Read the model definition and answer for the solid it produces. Units are mm, in the model's axes. A direction names the side the tool comes from. Round coordinates to 2 decimals unless told otherwise and drop trailing zeros. Order: outer loops, then holes, each group sorted by start corner. A loop starts at its lowest first (then second) coordinate and runs counter-clockwise, first axis right, second up. Notation, with made-up numbers: (38, -38.5) - (58, -38.5) arc R17 ccw to (58, -28.5) - close; hole circle Ø3 at (14.5, 23). An arc over 180 degrees is marked (long way). One line per question, with ' | ' between items. Start each with the question number.
1) For faces 1 (the flat face through (0, 1, 0)), 2 (the flat face through (14, -37, 12)), determine the directions among +Z, -Z, +X, -X, +Y, -Y from which every point of the face is accessible in a straight line to the end or side of a thin tool.
2) The part is cut by section D-D, the plane z = 20. Count the separate pieces of the cut face and the enclosed holes in it, plus the area to 3 significant figures.
3) Straight lines are drawn through the part: line 1 (Y direction, x = 16.5, z = 17.25); line 2 (X direction, y = -36.5, z = 6.5); line 3 (Y direction, x = -17.5, z = 22.5). For each, find the intervals that lie inside material, in ascending order. Write a range as from..to.
4) Flat-ended cylindrical pins translate along their axes: pin 1 (4 mm diameter, centred on x = -6.5, y = -4, fed in from +Z); pin 2 (1.2 mm diameter, centred on x = -16.5, y = -36, fed in from +Z). Find the tip coordinate at first contact, or state that the pin passes through.
5) The part is cut by section C-C, the plane y = 36.5. Give the vertices of the cut face in (x, z).
6) The part is cut by section B-B, the plane x = 0. Give the vertices of the cut face in (y, z), plus the area to 3 significant figures.
7) The mould has two halves that part along X. Classify faces 3 (the flat face through (-20, -1, 12)), 4 (the flat face through (-19.4, 0.2, 25)), 5 (the flat face through (16, 38, 23)): pulls with the +X half, pulls with the -X half, needs draft (parallel to the pull), parting line crosses it, or undercut.
8) The part is cut by section A-A, the plane z = 4.75. Give the vertices of the cut face in (x, y).
from build123d import *

# Parameters (mm, degrees)
F0_W     = 40
F0_H     = 80
F1_DEPTH = 25
F2_T     = -1
F3_W     = 5
F3_H     = 5
F3_R     = 0.75
F3_W_2   = 3
F3_H_2   = 1
F4_DEPTH = 22
F6_DEPTH = 25


with BuildPart() as f1:
    # F0 (on Top) → F1 (new body)
    with BuildSketch(Plane.XY):
        Rectangle(F0_W, F0_H)
    extrude(amount=F1_DEPTH)

    # F2
    f2_openings = [f1.faces().sort_by_distance(p)[0] for p in [
        (0, 0, 25),
    ]]
    offset(amount=F2_T, openings=f2_openings)

    # F3 (on face) → F4 (join)
    with BuildSketch(Plane.XY.offset(1)):
        with Locations((-16.5, 36.5)):
            Rectangle(F3_W, F3_H)
        with Locations((-16.5, 36.5)):
            Circle(F3_R, mode=Mode.SUBTRACT)
        with Locations((-16.5, -36.5)):
            Rectangle(F3_W, F3_H)
        with Locations((-16.5, -36.5)):
            Circle(F3_R, mode=Mode.SUBTRACT)
        with Locations((16.5, 36.5)):
            Rectangle(F3_W, F3_H)
        with Locations((16.5, 36.5)):
            Circle(F3_R, mode=Mode.SUBTRACT)
        with Locations((16.5, -36.5)):
            Rectangle(F3_W, F3_H)
        with Locations((16.5, -36.5)):
            Circle(F3_R, mode=Mode.SUBTRACT)
        with Locations((-17.5, 0)):
            Rectangle(F3_W_2, F3_H_2)
        with Locations((17.5, 0)):
            Rectangle(F3_W_2, F3_H_2)
    extrude(amount=F4_DEPTH)

    # F5 (on face) → F6 (cut)
    with BuildSketch(Plane.XZ.offset(40)):
        with BuildLine():
            Line((2, 25), (-2, 25))
            Line((-2, 25), (-2, 21))
            ThreePointArc((-2, 21), (0, 19), (2, 21))
            Line((2, 21), (2, 25))
        make_face()
    extrude(amount=-F6_DEPTH, mode=Mode.SUBTRACT)


solid = f1.part
Values:
1) face 1: -Z, +X, -X, +Y, -Y | face 2: +Z
2) separate pieces: 1 | enclosed holes: 4 | area: 331 mm^2
3) line 1: y = -40..-37.25, -35.75..-34, -0.5..0.5, 34..35.75, 37.25..40 | line 2: x = -20..-17.25, -15.75..-14, 14..15.75, 17.25..20 | line 3: y = -40..-34, -0.5..0.5, 34..40
4) pin 1: stops at z = 1 | pin 2: stops at z = 23
5) outline: (-20, 0) - (20, 0) - (20, 25) - (19, 25) - (19, 23) - (17.25, 23) - (17.25, 1) - (15.75, 1) - (15.75, 23) - (14, 23) - (14, 1) - (-14, 1) - (-14, 23) - (-15.75, 23) - (-15.75, 1) - (-17.25, 1) - (-17.25, 23) - (-19, 23) - (-19, 25) - (-20, 25) - close
6) outline: (-40, 0) - (40, 0) - (40, 25) - (39, 25) - (39, 1) - (-39, 1) - (-39, 19) - (-40, 19) - close | area: 122 mm^2
7) face 3: pulls with the -X half | face 4: needs draft | face 5: undercut
8) outline: (-20, -40) - (20, -40) - (20, 40) - (-20, 40) - close; hole (-19, -34) - (-14, -34) - (-14, -39) - (14, -39) - (14, -34) - (19, -34) - (19, -0.5) - (16, -0.5) - (16, 0.5) - (19, 0.5) - (19, 34) - (14, 34) - (14, 39) - (-14, 39) - (-14, 34) - (-19, 34) - (-19, 0.5) - (-16, 0.5) - (-16, -0.5) - (-19, -0.5) - close; hole circle Ø1.5 at (-16.5, -36.5); hole circle Ø1.5 at (-16.5, 36.5); hole circle Ø1.5 at (16.5, -36.5); hole circle Ø1.5 at (16.5, 36.5)
